Design review of the part built by this model. Coordinates are the model's own, in mm. Round coordinates to 2 decimals unless told otherwise and drop trailing zeros. Loops run counter-clockwise (first coordinate to the right, second up) from the corner with the lowest first, then second, coordinate; pieces in that order, holes last. Notation, with made-up numbers: M 77.25,52 L 85.25,52 A29 ccw 85.25,90 Z; hole C 39.25,6 d2. An arc over 180 degrees is marked long. One line per item, written item: value. Start each with the question number.
Item 1: For line 1 along X through (y, z) = (3, 2.5); line 2 along Z through (x, y) = (7.5, 5.75); line 3 along Z through (x, y) = (8, 3), list the stretches that pass through material, from the lowest coordinate up.
Item 2: We need section C-C (x = -46). Write out the cut boundary in (y, z).
Item 3: Mouldability with a two-part tool opening along Z and no side actions: class faces 1 (the flat face through (-64.84, 3.13, 37.69)), 2 (the cylindrical face through (-24.92, 3.22, -51.74)), 3 (the flat face through (-44.8, 3.1, -24.9)) as released by +Z, released by -Z, zero draft, split by the parting line, or undercut.
Item 4: Clearance check with flat-ended pins moving along their axes: pin 1 (4 mm diameter, centred on x = 30.1, z = 46.25, fed in from +Y); pin 2 (1.5 mm diameter, centred on y = 2.5, z = 12, fed in from +X). State where each tip first meets the part, or that it passes through.
Item 5: We need section A-A (y = 2). State how many separate pieces and enclosed holes the cut face has, then the cut area to 3 significant figures.
Item 6: We need section B-B (z = -21). Write out the cut boundary in (x, y).
from build123d import *

# Parameters (mm, degrees)
BOSS_EXTRUDE1_DEPTH = 6.35
SKETCH9_R           = 2.6
CUT_EXTRUDE1_DEPTH  = 105.776848123
SKETCH12_R          = 2.6
CUT_EXTRUDE4_DEPTH  = 105.776848123


with BuildPart() as part:
    # Sketch1 → Boss-Extrude1 (new body)
    with BuildSketch(Plane(origin=(0, 0, 0), x_dir=(1, 0, 0), z_dir=(0, 1, 0))):
        Polygon((-15.875, 75), (15.875, 75), (72.889405284, -23.751846715), (57.014405284, -51.248153285), (-57.014405284, -51.248153285), (-72.889405284, -23.751846715), align=None)
    extrude(amount=BOSS_EXTRUDE1_DEPTH)

    # Sketch9 → Cut-Extrude1 (cut, through all)
    with BuildSketch(Plane(origin=(0, 6.35, 0), x_dir=(1, 0, 0), z_dir=(0, 1, 0))):
        with Locations(Location((-25.030312278, 49.142819263, 0), (0, 0, 270))):
            Circle(SKETCH9_R)
        with Locations(Location((25.008570083, 49.180192562, 0), (0, 0, 270))):
            Circle(SKETCH9_R)
        with Locations(Location((55.008731986, -2.78123819, 0), (0, 0, 270))):
            Circle(SKETCH9_R)
        with Locations(Location((30.09884337, -46.248153285, 0), (0, 0, 270))):
            Circle(SKETCH9_R)
        with Locations(Location((-55.030188745, -2.818776286, 0), (0, 0, 270))):
            Circle(SKETCH9_R)
        with Locations(Location((-29.90115663, -46.248153285, 0), (0, 0, 270))):
            Circle(SKETCH9_R)
    extrude(amount=-CUT_EXTRUDE1_DEPTH, mode=Mode.SUBTRACT)

    # Sketch12 → Cut-Extrude4 (cut, through all)
    with BuildSketch(Plane(origin=(0, 6.35, 0), x_dir=(1, 0, 0), z_dir=(0, 1, 0))):
        with Locations(Location((33.539251883, -19.363896103, 0), (0, 0, 270))):
            Circle(SKETCH12_R)
        with Locations(Location((7.55848977, -4.363896103, 0), (0, 0, 270))):
            Circle(SKETCH12_R)
        with Locations(Location((-19.638606793, 11.338354919, 0), (0, 0, 270))):
            Circle(SKETCH12_R)
    extrude(amount=-CUT_EXTRUDE4_DEPTH, mode=Mode.SUBTRACT)


solid = part.part
A:
1. line 1: -60.62 to -57.61, -52.45 to 5.75, 9.37 to 52.42, 57.59 to 60.62
1. line 2: -75 to 1.76, 6.96 to 51.25
1. line 3: -75 to 1.8, 6.93 to 51.25
2. outline: M 0,-22.82 L 6.35,-22.82 L 6.35,51.25 L 0,51.25 Z
3. face 1: released by +Z
3. face 2: undercut
3. face 3: released by -Z
4. pin 1: through
4. pin 2: x = 66.54
5. separate pieces: 1
5. enclosed holes: 9
5. area: 12,100 mm2
6. outline: M -47.05,0 L 47.05,0 L 47.05,6.35 L -47.05,6.35 Z
